Source: CAD feature listing. Evaluate the final solid. Frame: model axes, mm. A direction names the side the tool comes from. Round coordinates to 2 decimals unless told otherwise and drop trailing zeros. Order: outer loops, then holes, each group sorted by start corner. A loop starts at its lowest first (then second) coordinate and runs counter-clockwise, first axis right, second up. Notation, with made-up numbers: (-1, 37.5) -> (13, 37.5) arc R11 ccw to (13, 50.5) -> close; hole circle Ø1 at (1, 8.25). An arc over 180 degrees is marked (long way). Answer as CSV lines item,"result".
from build123d import *

# Parameters (mm, degrees)
SKETCH1_W            = 137
SKETCH1_H            = 100
BOSS_EXTRUDE1_DEPTH  = 2
BOSS_EXTRUDE2_DEPTH  = 2
SKETCH4_W            = 135
SKETCH4_H            = 40
BOSS_EXTRUDE3_DEPTH  = 2
BOSS_EXTRUDE6_START  = -22.5
BOSS_EXTRUDE6_DEPTH  = 2
BOSS_EXTRUDE7_START  = -45
BOSS_EXTRUDE7_DEPTH  = 2
BOSS_EXTRUDE8_START  = -67.5
BOSS_EXTRUDE8_DEPTH  = 2
BOSS_EXTRUDE9_START  = -90
BOSS_EXTRUDE9_DEPTH  = 2
BOSS_EXTRUDE10_START = -112.5
BOSS_EXTRUDE10_DEPTH = 2
BOSS_EXTRUDE11_START = -135
BOSS_EXTRUDE11_DEPTH = 2
BOSS_EXTRUDE12_DEPTH = 133


with BuildPart() as part:
    # Sketch1 → Boss-Extrude1 (new body)
    with BuildSketch(Plane(origin=(0, 0, 0), x_dir=(1, 0, 0), z_dir=(0, 1, 0))):
        with Locations((68.5, 50)):
            Rectangle(SKETCH1_W, SKETCH1_H)
    extrude(amount=BOSS_EXTRUDE1_DEPTH)

    # Sketch3 → Boss-Extrude2 (add)
    with BuildSketch(Plane.ZY):
        Polygon((-100, 2), (-100, 42), (-20, 42), (0, 22), (0, 2), align=None)
    extrude(amount=-BOSS_EXTRUDE2_DEPTH)

    # Sketch4 → Boss-Extrude3 (add)
    with BuildSketch(Plane(origin=(0, 0, -100), x_dir=(-1, 0, 0), z_dir=(0, 0, -1))):
        with Locations((-69.5, 22)):
            Rectangle(SKETCH4_W, SKETCH4_H)
    extrude(amount=-BOSS_EXTRUDE3_DEPTH)

    # Sketch3<5> → Boss-Extrude6 (add)
    with BuildSketch(Plane.ZY.offset(BOSS_EXTRUDE6_START)):
        Polygon((-100, 2), (-100, 42), (-20, 42), (0, 22), (0, 2), align=None)
    extrude(amount=-BOSS_EXTRUDE6_DEPTH)

    # Sketch3<6> → Boss-Extrude7 (add)
    with BuildSketch(Plane.ZY.offset(BOSS_EXTRUDE7_START)):
        Polygon((-100, 2), (-100, 42), (-20, 42), (0, 22), (0, 2), align=None)
    extrude(amount=-BOSS_EXTRUDE7_DEPTH)

    # Sketch3<7> → Boss-Extrude8 (add)
    with BuildSketch(Plane.ZY.offset(BOSS_EXTRUDE8_START)):
        Polygon((-100, 2), (-100, 42), (-20, 42), (0, 22), (0, 2), align=None)
    extrude(amount=-BOSS_EXTRUDE8_DEPTH)

    # Sketch3<8> → Boss-Extrude9 (add)
    with BuildSketch(Plane.ZY.offset(BOSS_EXTRUDE9_START)):
        Polygon((-100, 2), (-100, 42), (-20, 42), (0, 22), (0, 2), align=None)
    extrude(amount=-BOSS_EXTRUDE9_DEPTH)

    # Sketch3<9> → Boss-Extrude10 (add)
    with BuildSketch(Plane.ZY.offset(BOSS_EXTRUDE10_START)):
        Polygon((-100, 2), (-100, 42), (-20, 42), (0, 22), (0, 2), align=None)
    extrude(amount=-BOSS_EXTRUDE10_DEPTH)

    # Sketch3<10> → Boss-Extrude11 (add)
    with BuildSketch(Plane.ZY.offset(BOSS_EXTRUDE11_START)):
        Polygon((-100, 2), (-100, 42), (-20, 42), (0, 22), (0, 2), align=None)
    extrude(amount=-BOSS_EXTRUDE11_DEPTH)

    # Sketch5 → Boss-Extrude12 (add)
    with BuildSketch(Plane(origin=(2, 0, 0), x_dir=(0, 0, -1), z_dir=(1, 0, 0))):
        Polygon((0, 2), (0, 6.5), (6.5, 6.5), (11, 2), align=None)
    extrude(amount=BOSS_EXTRUDE12_DEPTH)


solid = part.part
1. Section query B-B on x = 98.5. Return loops of the section in (y, z).
Results below:
outline,"(0, -100) -> (42, -100) -> (42, -98) -> (2, -98) -> (2, -11) -> (6.5, -6.5) -> (6.5, 0) -> (0, 0) -> close"
2. Pin query (flat end, axial travel): pin 1 (3 mm diameter, centred on x = 128.5, z = -3.5, fed in from +Y); pin 2 (4 mm diameter, centred on x = 58, y = 36.5, fed in from +Z). Return the tip coordinate at first contact, or that it passes through.
Results below:
pin 1,"y = 6.5"
pin 2,"z = -98"
3. Section query A-A on y = 36. Return loops of the section in (x, z), and give its area (3 significant figures).
Results below:
outline,"(0, -100) -> (137, -100) -> (137, -14) -> (135, -14) -> (135, -98) -> (114.5, -98) -> (114.5, -14) -> (112.5, -14) -> (112.5, -98) -> (92, -98) -> (92, -14) -> (90, -14) -> (90, -98) -> (69.5, -98) -> (69.5, -14) -> (67.5, -14) -> (67.5, -98) -> (47, -98) -> (47, -14) -> (45, -14) -> (45, -98) -> (24.5, -98) -> (24.5, -14) -> (22.5, -14) -> (22.5, -98) -> (2, -98) -> (2, -14) -> (0, -14) -> close"
area,"1,450 mm2"
4. Section query C-C on z = -83.5. Return loops of the section in (x, y), and give its area (3 significant figures).
Results below:
outline,"(0, 0) -> (137, 0) -> (137, 42) -> (135, 42) -> (135, 2) -> (114.5, 2) -> (114.5, 42) -> (112.5, 42) -> (112.5, 2) -> (92, 2) -> (92, 42) -> (90, 42) -> (90, 2) -> (69.5, 2) -> (69.5, 42) -> (67.5, 42) -> (67.5, 2) -> (47, 2) -> (47, 42) -> (45, 42) -> (45, 2) -> (24.5, 2) -> (24.5, 42) -> (22.5, 42) -> (22.5, 2) -> (2, 2) -> (2, 42) -> (0, 42) -> close"
area,"834 mm2"
5. Mould query, pull axis X, two halves, no side actions, for faces 1 (the flat face through (92, 22, -48)), 2 (the flat face through (91, 32, -10)), 3 (the flat face through (137, 21, -51)). Classes: released by +X, released by -X, zero draft, split by the parting line, or undercut.
Results below:
face 1,"undercut"
face 2,"zero draft"
face 3,"released by +X"
6. Line query: L1, parallel to Z at x = 49.5, y = 40; L2, parallel to Y at x = 94.5, z = -29; L3, parallel to Z at x = 23, y = 33. Output: solid intervals per line, ascending. Write a range as [from, to].
Results below:
L1,"[-100, -98]"
L2,"[0, 2]"
L3,"[-100, -11]"
7. Reachability of faces 4 (the flat face through (35, 2, -55)), 5 (the flat face through (35, 6.5, -3)), 6 (the flat face through (46, 32, -10)) from +Z, -Z, +X, -X, +Y, -Y: full face, straight path, thin tool, end or side. Return the list, or none.
Results below:
face 4,"+Y"
face 5,"+Z, +Y"
face 6,"+Z, +X, -X, +Y"
